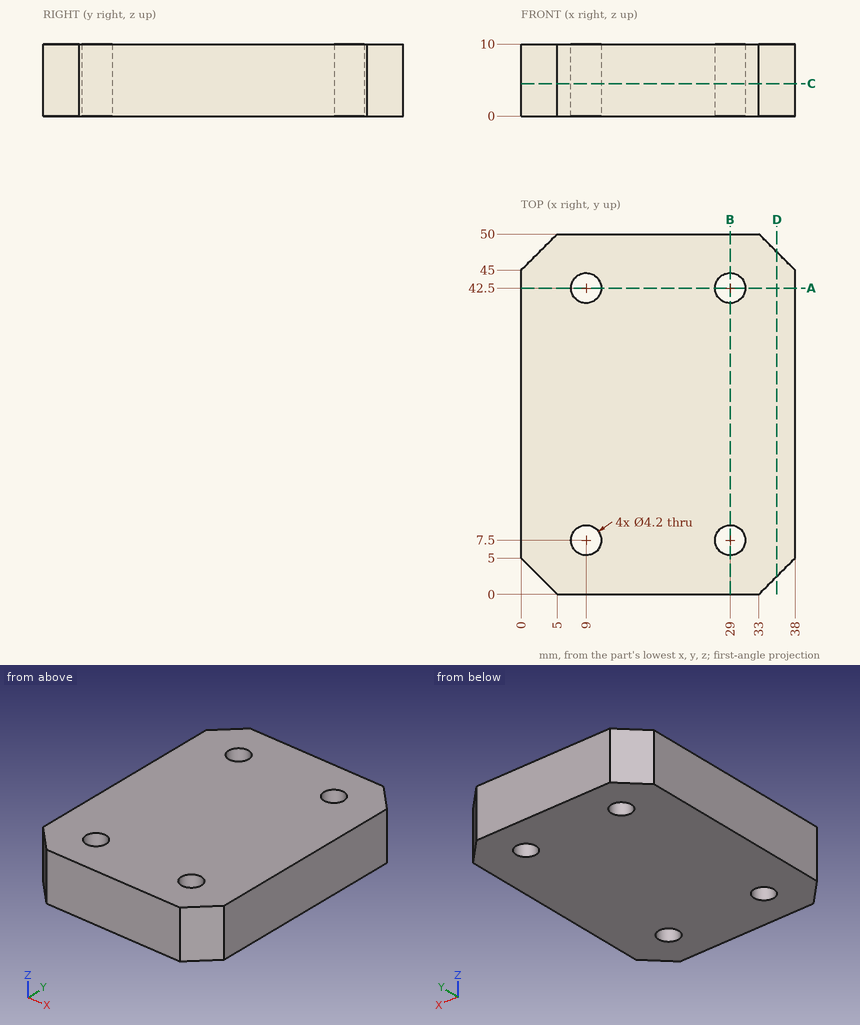
Source: three-view drawing plus pictorial views. Frame: mm from the lowest corner of the part. Round coordinates to 2 decimals unless told otherwise and drop trailing zeros. Loops run counter-clockwise (first coordinate to the right, second up) from the corner with the lowest first, then second, coordinate; pieces in that order, holes last.
1. Section query B-B on x = 29. Output: boundary loops of the cut face in (y, z), and give its area (3 significant figures).
2. Section query D-D on x = 35.5. Output: boundary loops of the cut face in (y, z), and give its area (3 significant figures).
3. Section query A-A on y = 42.5. Output: boundary loops of the cut face in (x, z), and give its area (3 significant figures).
4. Contact query for a flat-ended pin moving along its axis: pin 1 (3.5 mm diameter, centred on x = 29, y = 42.5, fed in from -Z). Output: stop coordinate, or through.
5. Ray query, L1, parallel to Y at x = 9, z = 6; L2, parallel to Y at x = 28.5, z = 3.5; L3, parallel to Y at x = 36, z = 1. Return the intervals inside material, ascending.
6. Section query C-C on z = 4.5. Output: boundary loops of the cut face in (x, y), and give its area (3 significant figures).
Answers below:
1. outline: (0, 0) - (5.4, 0) - (5.4, 10) - (0, 10) - close; (9.6, 0) - (40.4, 0) - (40.4, 10) - (9.6, 10) - close; (44.6, 0) - (50, 0) - (50, 10) - (44.6, 10) - close
1. area: 416 mm2
2. outline: (2.5, 0) - (47.5, 0) - (47.5, 10) - (2.5, 10) - close
2. area: 450 mm2
3. outline: (0, 0) - (6.9, 0) - (6.9, 10) - (0, 10) - close; (11.1, 0) - (26.9, 0) - (26.9, 10) - (11.1, 10) - close; (31.1, 0) - (38, 0) - (38, 10) - (31.1, 10) - close
3. area: 296 mm2
4. pin 1: passes through
5. L1: y = 0 to 5.4, 9.6 to 40.4, 44.6 to 50
5. L2: y = 0 to 5.46, 9.54 to 40.46, 44.54 to 50
5. L3: y = 3 to 47
6. outline: (0, 5) - (5, 0) - (33, 0) - (38, 5) - (38, 45) - (33, 50) - (5, 50) - (0, 45) - close; hole circle Ø4.2 at (9, 7.5); hole circle Ø4.2 at (9, 42.5); hole circle Ø4.2 at (29, 7.5); hole circle Ø4.2 at (29, 42.5)
6. area: 1,790 mm2
